Can you work these out from the model? Positions are in its coordinate system, mm. A direction names the side the tool comes from. Coordinates: 2 decimals unless noted, no trailing zeros. Order: outer loops, then holes, each group sorted by start corner. A loop starts at its lowest first (then second) coordinate and runs counter-clockwise, first axis right, second up. Notation, with made-up numbers: (-23, -21.5) -> (28, -21.5) arc R17 cw to (28, 1.5) -> close; hole circle Ø10 at (5.25, -13). An arc over 180 degrees is marked (long way). Return JSON: item names as keys, results as strings. Group by question number.
1) For pin 1 (2 mm diameter, centred on x = -1, z = 3, fed in from +Y); pin 2 (2 mm diameter, centred on x = 1.5, z = 6, fed in from -Y); pin 3 (1 mm diameter, centred on y = -1.5, z = -0.5, fed in from -X), each with a flat end and sliding along its axis, tell me the tip position at first contact or that it passes through.
2) For faces 5 (the cylindrical face through (-0.338, 2.578, 4.198)), 6 (the flat face through (0, 0, -0.5)), 7 (the cylindrical face through (3.233, -1.341, 0.007)), which set-ups out of +Z, -Z, +X, -X, +Y, -Y let a thin tool reach every point of the face, with its end or its side?
3) If we section it at C-C, the plane z = 2.5: Please give me the cut outline in (x, y).
4) Thinking about a two-plate mould opening in Y: for faces 1 (the cylindrical face through (2.003, -0.631, -2.226)), 2 (the cylindrical face through (2.003, 0.631, 4.198)), 3 (the cylindrical face through (-0.338, -2.578, -2.226)), 4 (the flat face through (0, 3, -0.5)), which applies, +Y half, -Y half, draft (parallel to the pull), parting line (faces both ways), or undercut?
5) If I drill on probe 1 along Y at (x, z) = (0, 3); probe 2 along X at (y, z) = (1.25, -0.75), over which ranges is the centre line in solid material (lowest first)? Write a range as from..to.
6) If we section it at A-A, the plane y = 0: Please give me the cut outline in (x, z).
7) If we section it at B-B, the plane x = -1.25: Please give me the cut outline in (y, z), then the cut area to 3 significant figures.
from build123d import *

# Parameters (mm, degrees)
F0_R     = 3.5
F1_DEPTH = 0.5
F2_R     = 2.6
F2_R_2   = 2.1
F3_DEPTH = 7.5
F4_R     = 2.6
F4_R_2   = 2.1
F5_DEPTH = 3.5


with BuildPart() as f1:
    # F0 (on Top) → F1 (new body, symmetric)
    with BuildSketch(Plane.XY):
        Circle(F0_R)
    extrude(amount=F1_DEPTH, both=True)

    # F2 (on face) → F3 (join)
    with BuildSketch(Plane.XY.offset(0.5)):
        Circle(F2_R)
        Circle(F2_R_2, mode=Mode.SUBTRACT)
    extrude(amount=F3_DEPTH)

    # F4 (on face) → F5 (join)
    with BuildSketch(Plane(origin=(0, 0, -0.5), x_dir=(1, 0, 0), z_dir=(0, 0, -1))):
        Circle(F4_R)
        Circle(F4_R_2, mode=Mode.SUBTRACT)
    extrude(amount=F5_DEPTH)


solid = f1.part
Result sheet:
{
 "1": {"pin 1": "stops at y = 2.6", "pin 2": "stops at y = -2.55", "pin 3": "stops at x = -3.35"},
 "2": {"face 5": "+Z", "face 6": "-Z", "face 7": "+Z, -Z"},
 "3": {"outline": "circle Ø5.2 at (0, 0); hole circle Ø4.2 at (0, 0)"},
 "4": {"face 1": "undercut", "face 2": "undercut", "face 3": "parting line", "face 4": "draft"},
 "5": {"probe 1": "y = -2.6..-2.1, 2.1..2.6", "probe 2": "x = -2.28..-1.69, 1.69..2.28"},
 "6": {"outline": "(-3.5, -0.5) -> (-2.6, -0.5) -> (-2.6, -4) -> (-2.1, -4) -> (-2.1, -0.5) -> (2.1, -0.5) -> (2.1, -4) -> (2.6, -4) -> (2.6, -0.5) -> (3.5, -0.5) -> (3.5, 0.5) -> (2.6, 0.5) -> (2.6, 8) -> (2.1, 8) -> (2.1, 0.5) -> (-2.1, 0.5) -> (-2.1, 8) -> (-2.6, 8) -> (-2.6, 0.5) -> (-3.5, 0.5) -> close"},
 "7": {"outline": "(-3.27, -0.5) -> (-2.28, -0.5) -> (-2.28, -4) -> (-1.69, -4) -> (-1.69, -0.5) -> (1.69, -0.5) -> (1.69, -4) -> (2.28, -4) -> (2.28, -0.5) -> (3.27, -0.5) -> (3.27, 0.5) -> (2.28, 0.5) -> (2.28, 8) -> (1.69, 8) -> (1.69, 0.5) -> (-1.69, 0.5) -> (-1.69, 8) -> (-2.28, 8) -> (-2.28, 0.5) -> (-3.27, 0.5) -> close", "area": "19.6 mm2"}
}
